Check sheet for the modelled part. Datum: model origin and axes. Units: mm. Face numbers are marked on the shaded views. A direction names the side the tool comes from. Give positions to 0.01 mm unless a question says otherwise; leave off trailing zeros. Order: outer loops, then holes, each group sorted by start corner. A loop starts at its lowest first (then second) coordinate and runs counter-clockwise, first axis right, second up. Notation, with made-up numbers: (18.25, 35) -> (58.25, 35) arc R10 cw to (58.25, 50) -> close; hole circle Ø11 at (88.25, -26). An arc over 180 degrees is marked (long way). Write each question's results on one line, items separated by ' | '.
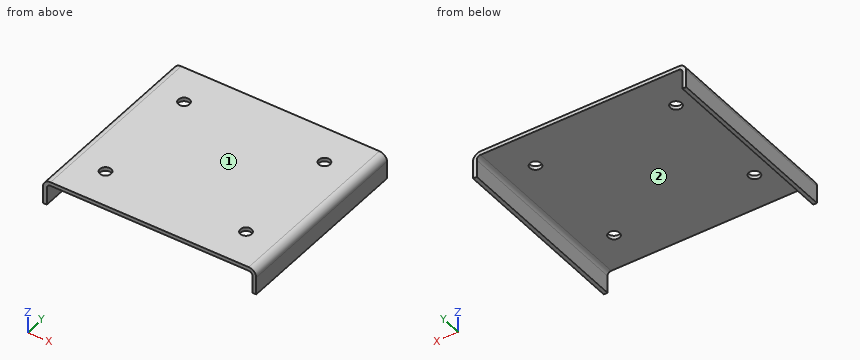
Autodesk Inventor part; units mm, degrees
ref_plane "YZ Plane" through (0, 0, 0) normal (1, 0, 0) x (0, 1, 0)
ref_plane "XZ Plane" through (0, 0, 0) normal (0, 1, 0) x (-1, 0, 0)
ref_plane "XY Plane" through (0, 0, 0) normal (0, 0, 1) x (1, 0, 0)
sketch "Sketch1" plane through (0, 0, 0) normal (0, 0, 1) x (1, 0, 0)
  line L0 (85, -75) -> (-85, -75)
  line L1 (-85, -75) -> (-85, 75)
  line L2 (-85, 75) -> (85, 75)
  line L3 (85, 75) -> (85, -75)
  line L4 (85, 75) -> (-85, -75) construction
  point P0 (0, 0)
  point P1 (0, 0)
  dimension "d1" = 150
  dimension "d2" = 170
extrude "Plate1" add sketch "Sketch1" along normal blind 3
sketch "Sketch2" plane through (0, 0, 0) normal (0, 0, 1) x (1, 0, 0)
  line L0 (56, -45) -> (-56, -45) construction
  line L1 (-56, -45) -> (-56, 45) construction
  line L2 (-56, 45) -> (56, 45) construction
  line L3 (56, 45) -> (56, -45) construction
  line L4 (56, -45) -> (-56, 45) construction
  line L5 (-56, -45) -> (56, 45) construction
  circle A0 centre (-56, -45) radius 4.5
  circle A1 centre (56, -45) radius 4.5
  circle A2 centre (56, 45) radius 4.5
  circle A3 centre (-56, 45) radius 4.5
  line L6 (56, 0) -> (-56, 0) construction
  point P0 (0, 0)
  point P1 (0, 0)
  dimension "d4" = 112
  dimension "d5" = 90
  dimension "d7" = 9
extrude "Extrusion1" cut sketch "Sketch2" along normal through all
sketch "Sketch3" plane through (-82, 75, 3) normal (-1, 0, 0) x (0, -1, 0)
  line L0 (150, 0) -> (0, 0)
  line L1 (0, 0) -> (0, -20)
  line L2 (0, -20) -> (150, -20)
  line L3 (150, -20) -> (150, 0)
edge flange "Flange1" height 20 angle 90 thickness 3 bend radius 3 thickness toward (-1, 0, 0) relief tear relief width 3 relief depth 1.5 corner gap 3 corner form 0 edges at (-85, 0, 0) (85, 0, 0) wall of the first edge with corners at (-82, -75, 3) (-82, 75, 3) (-82, 75, -17) (-82, -75, -17)
bend "Bend1"
corner "Corner1"
sketch "Sketch4" plane through (0, 0, 0) normal (0, 0, 1) x (1, 0, 0)
  circle A0 centre (0, 75) radius 17.5
  line L0 (0, 125) -> (0, 105) construction
  line L1 (-3, 125) -> (-3, 105)
  line L2 (3, 105) -> (3, 125)
  arc A1 (3, 125) -> (-3, 125) centre (0, 125) ccw
  arc A2 (-3, 105) -> (3, 105) centre (0, 105) ccw
  arc A3 (34.641, 95) -> (20, 109.641) centre (0, 75) ccw construction
  arc A4 (37.2391, 96.5) -> (21.5, 112.2391) centre (0, 75) ccw
  arc A5 (32.0429, 93.5) -> (18.5, 107.0429) centre (0, 75) ccw
  arc A6 (32.0429, 93.5) -> (37.2391, 96.5) centre (34.641, 95) ccw
  arc A7 (21.5, 112.2391) -> (18.5, 107.0429) centre (20, 109.641) ccw
  line L3 (0, 75) -> (20, 109.641) construction
  line L4 (0, 75) -> (40, 75) construction
  line L5 (0, 75) -> (34.641, 95) construction
  point P0 (0, 0)
  point P1 (0, 115)
  dimension "d20" = 20
  dimension "d21" = 6
  dimension "d22" = 30
  dimension "d23" = 60
  dimension "d24" = 30
  dimension "d25" = 6
  dimension "d26" = 40
extrude "Extrusion2" [suppressed]
pattern_circular "Circular Pattern1" [suppressed]
equation "\"d0\" = Thickness"
equation "\"d10\" = BendReliefWidth"
equation "\"d11\" = BendReliefDepth"
equation "\"d12\" = MinimumRemnant"
equation "\"d13\" = TransitionRadius"
equation "\"d16\" = BendRadius"
equation "\"d17\" = CornerReliefSize"
equation "\"d18\" = GapSize"
equation "\"d19\" = JacobiRadiusSize"
equation "\"BendRadius\" = Thickness"
equation "\"BendReliefWidth\" = Thickness"
equation "\"BendReliefDepth\" = 0.5 * Thickness"
equation "\"CornerReliefSize\" = 4 * Thickness"
equation "\"MinimumRemnant\" = 2 * Thickness"
equation "\"TransitionRadius\" = BendRadius"
equation "\"JacobiRadiusSize\" = BendRadius"
equation "\"GapSize\" = Thickness"
properties part number "GNH 026  Motor pillar 2" material "Stainless Steel"
1. Gauge pin test, flat end, axial feed: pin 1 Ø2 at (x, y) = (-14, 20) entering from -Z. Record the tip position at first contact, or that the pin passes through.
Verdict:
pin 1: stops at z = 0
2. Section check A-A on z = -8. Record the cut outline in (x, y).
Verdict:
outline: (-85, -75) -> (-82, -75) -> (-82, 75) -> (-85, 75) -> close; (82, -75) -> (85, -75) -> (85, 75) -> (82, 75) -> close
3. Section check B-B on y = -45. Record the cut outline in (x, z).
Verdict:
outline: (-85, -17) -> (-82, -17) -> (-82, -3) arc R3 cw to (-79, 0) -> (-60.5, 0) -> (-60.5, 3) -> (-79, 3) arc R6 ccw to (-85, -3) -> close; (-51.5, 0) -> (51.5, 0) -> (51.5, 3) -> (-51.5, 3) -> close; (60.5, 0) -> (79, 0) arc R3 cw to (82, -3) -> (82, -17) -> (85, -17) -> (85, -3) arc R6 ccw to (79, 3) -> (60.5, 3) -> close
4. Section check C-C on x = -56. Record the cut outline in (y, z).
Verdict:
outline: (-75, 0) -> (-49.5, 0) -> (-49.5, 3) -> (-75, 3) -> close; (-40.5, 0) -> (40.5, 0) -> (40.5, 3) -> (-40.5, 3) -> close; (49.5, 0) -> (75, 0) -> (75, 3) -> (49.5, 3) -> close
5. Material ranges on probe 1 along Y at (x, z) = (-56, 1.65); probe 2 along X at (y, z) = (-16, -14.5); probe 3 along X at (y, z) = (45, 1.2), recorded low to high. Write a range as from..to.
Verdict:
probe 1: y = -75..-49.5, -40.5..40.5, 49.5..75 | probe 2: x = -85..-82, 82..85 | probe 3: x = -83.28..-60.5, -51.5..51.5, 60.5..83.28
6. Access from +Z, -Z, +X, -X, +Y, -Y to the whole of each face (thin tool, end or side, straight path). Record for the marked faces 1 and 2.
Verdict:
face 1: +Z, +X, -X, +Y, -Y | face 2: -Z, +Y, -Y
7. Section check D-D on y = 37.5. Record the cut outline in (x, z), then the cut area to 3 significant figures.
Verdict:
outline: (-85, -17) -> (-82, -17) -> (-82, -3) arc R3 cw to (-79, 0) -> (79, 0) arc R3 cw to (82, -3) -> (82, -17) -> (85, -17) -> (85, -3) arc R6 ccw to (79, 3) -> (-79, 3) arc R6 ccw to (-85, -3) -> close | area: 600 mm^2
